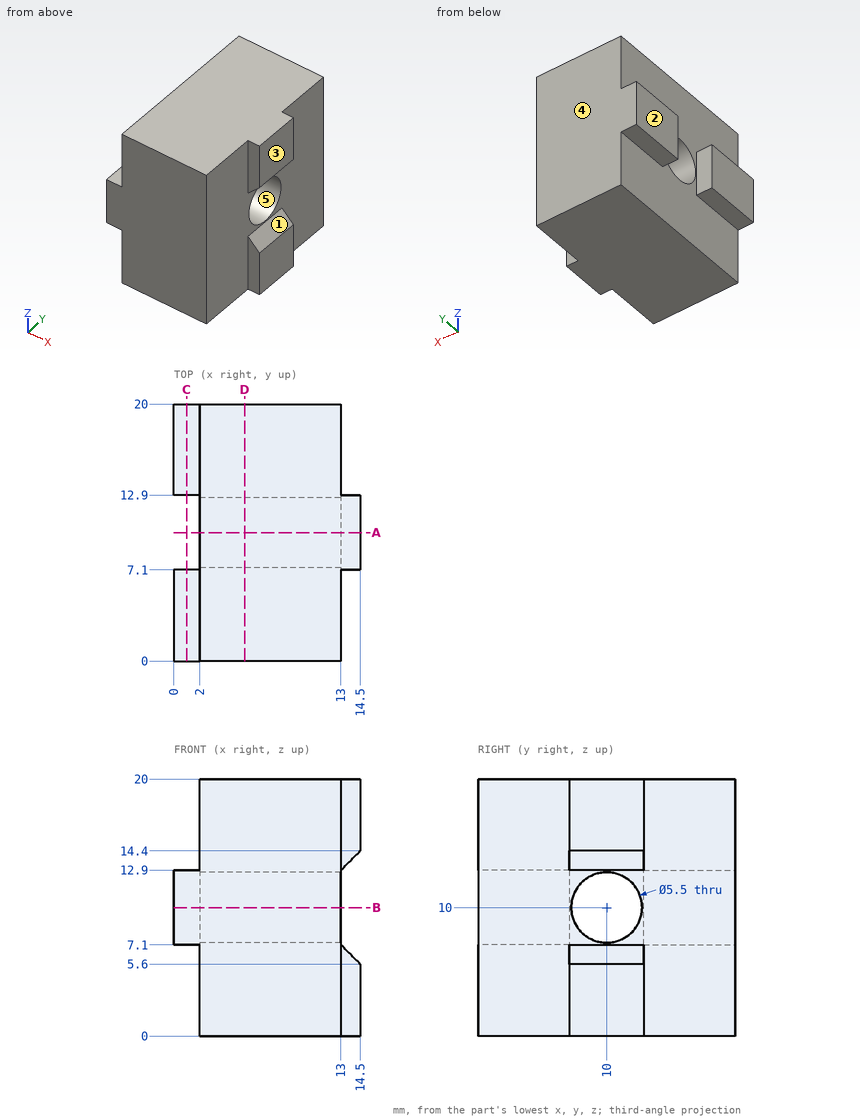
Verification items for this drawing (mm, ordinates from the low corner). A direction names the side the tool comes from. Coordinates: 2 decimals unless noted, no trailing zeros. Loops run counter-clockwise (first coordinate to the right, second up) from the corner with the lowest first, then second, coordinate; pieces in that order, holes last. Notation, with made-up numbers: (62.25, -12.5) -> (94.25, -12.5) arc R13 cw to (94.25, 8.5) -> close; hole circle Ø2 at (1, -29.75). An arc over 180 degrees is marked (long way). Answer in a Markdown table with one row per item. Add a question column.
1. Section check D-D, the plane x = 5.5. Enter the section's corners in (y, z), then the cut area to 3 significant figures.
2. Draft check along Y on the marked faces 3, 4 and 5. Enter one of: +Y half, -Y half, draft (parallel to the pull), parting line (faces both ways), or undercut.
3. Material ranges on probe 1 along Z at (x, y) = (7, 10); probe 2 along X at (y, z) = (4.25, 16), recorded low to high. Write a range as [from, to].
4. Section check B-B, the plane z = 10. Enter the section's corners in (x, y).
5. Section check A-A, the plane y = 10. Enter the section's corners in (x, z).
6. Access from +Z, -Z, +X, -X, +Y, -Y to the whole of each face (thin tool, end or side, straight path). Record for the marked faces 1 and 2.
7. Depth check by flat-ended pin: P1, Ø2, axis at y = 8, z = 18, coming from the -X side; P2, Ø0.8, axis at x = 14, z = 16.5, coming from the +Y side; P3, Ø1, axis at x = 1, y = 16, coming from the -Z side. Enter the tip coordinate at first touch or a pass-through.
8. Section check C-C, the plane x = 1. Enter the section's corners in (y, z), then the cut area to 3 significant figures.
Derived:
| question | item | result |
|---|---|---|
| 1 | outline | (0, 0) -> (20, 0) -> (20, 20) -> (0, 20) -> close; hole circle Ø5.5 at (10, 10) |
| 1 | area | 376 mm² |
| 2 | face 3 | draft |
| 2 | face 4 | +Y half |
| 2 | face 5 | undercut |
| 3 | probe 1 | z = [0, 7.25], [12.75, 20] |
| 3 | probe 2 | x = [2, 13] |
| 4 | outline | (0, 0) -> (13, 0) -> (13, 7.25) -> (2, 7.25) -> (2, 7.1) -> (0, 7.1) -> close; (0, 12.9) -> (2, 12.9) -> (2, 12.75) -> (13, 12.75) -> (13, 20) -> (0, 20) -> close |
| 5 | outline | (2, 0) -> (14.5, 0) -> (14.5, 5.6) -> (13, 7.1) -> (13, 7.25) -> (2, 7.25) -> close; (2, 12.75) -> (13, 12.75) -> (13, 12.9) -> (14.5, 14.4) -> (14.5, 20) -> (2, 20) -> close |
| 6 | face 1 | +X, +Y, -Y |
| 6 | face 2 | +Z, -Z, -X, +Y, -Y |
| 7 | P1 | stops at x = 2 |
| 7 | P2 | stops at y = 12.9 |
| 7 | P3 | stops at z = 7.1 |
| 8 | outline | (0, 7.1) -> (7.1, 7.1) -> (7.1, 12.9) -> (0, 12.9) -> close; (12.9, 7.1) -> (20, 7.1) -> (20, 12.9) -> (12.9, 12.9) -> close |
| 8 | area | 82.4 mm² |
